from build123d import *

# Parameters (mm, degrees)
SKETCH2_W                    = 10.4902
SKETCH2_H                    = 5.7531
SKETCH3_W                    = 3.0988
SKETCH3_H                    = 1.2446
SKETCH4_R                    = 3.1496
CUT_EXTRUDE1_DEPTH           = 8.89
SKETCH5_R                    = 1
BOSS_EXTRUDE1_DEPTH          = 7.62
FILLET1_R                    = 1
SKETCH6_W                    = 2.35
SKETCH6_H                    = 0.254
SKETCH6_W_2                  = 0.254
SKETCH6_H_2                  = 2.35
EXTRUDE_THIN1_DEPTH          = 4.4958
FILLET2_R                    = 1.1
F_0_75_0_75_DIAMETER_HOLE1_D = 0.75
F_0_75_0_75_DIAMETER_HOLE2_D = 0.75
SKETCH16_OUTSIDE_W           = 23.662
SKETCH16_OUTSIDE_H           = 23.662
SKETCH16_OUTSIDE_W_2         = 11.9888
SKETCH16_OUTSIDE_H_2         = 13.0048
CUT_EXTRUDE2_DEPTH           = 9.6012


with BuildPart() as part:
    # Sketch2 → Revolve1 (revolve)
    with BuildSketch(Plane(origin=(0, 0, 0), x_dir=(0, 0, -1), z_dir=(1, 0, 0)), mode=Mode.PRIVATE) as revolve1_sk:
        with BuildLine():
            Line((-2.0066, 0), (0, 0))
            Line((0, 0), (0, 5.7531))
            Line((0, 5.7531), (0, 6.9977))
            Line((0, 6.9977), (-1.2446, 6.9977))
            ThreePointArc((-1.2446, 6.9977), (-1.783415367, 6.774515367), (-2.0066, 6.2357))
            Line((-2.0066, 6.2357), (-2.0066, 0))
        make_face()
        with Locations((5.2451, 2.87655)):
            Rectangle(SKETCH2_W, SKETCH2_H)
    revolve(revolve1_sk.sketch.rotate(Axis((0, 0, 7.880629527), (0, 0, -1)), 90), axis=Axis((0, 0, 7.880629527), (0, 0, -1)))

    # Sketch4 → Cut-Extrude1 (cut)
    with BuildSketch(Plane.XY.offset(2.0066)):
        with Locations((0, -2.4511)):
            Circle(SKETCH4_R)
    extrude(amount=-CUT_EXTRUDE1_DEPTH, mode=Mode.SUBTRACT)


with BuildPart() as body_2:
    # Sketch3 → Revolve2 (revolve)
    with BuildSketch(Plane(origin=(0, 0, 0), x_dir=(0, 0, -1), z_dir=(1, 0, 0)), mode=Mode.PRIVATE) as revolve2_sk:
        with Locations((2.4384, 6.3754)):
            Rectangle(SKETCH3_W, SKETCH3_H)
        with BuildLine():
            ThreePointArc((0, 7.62), (0.111592316, 7.889407684), (0.381, 8.001))
            Line((0.381, 8.001), (0.508, 8.001))
            ThreePointArc((0.508, 8.001), (0.777407684, 7.889407684), (0.889, 7.62))
            Line((0.889, 7.62), (0.889, 5.7531))
            Line((0.889, 5.7531), (0, 5.7531))
            Line((0, 5.7531), (0, 7.62))
        make_face()
    revolve(revolve2_sk.sketch.rotate(Axis((0, 0, 6.77031441), (0, 0, -1)), 90), axis=Axis((0, 0, 6.77031441), (0, 0, -1)))


    add(part.part)  # Boss-Extrude1 merges part
    # Sketch5 → Boss-Extrude1 (add)
    with BuildSketch(Plane.XY.offset(-6.8834)):
        with Locations(Location((0, -2.4511, 0), (0, 0, 180))):
            Circle(SKETCH5_R)
    extrude(amount=BOSS_EXTRUDE1_DEPTH)

    # Fillet1
    fillet1_edges = [body_2.edges().sort_by_distance(p)[0] for p in [
        (1, -2.4511, 0.7366),
    ]]
    fillet(fillet1_edges, radius=FILLET1_R)

    # Sketch6 → Extrude-Thin1 (add)
    with BuildSketch(Plane(origin=(0, 0, -10.4902), x_dir=(-1, 0, 0), z_dir=(0, 0, -1))):
        with Locations((0, 4.010257453)):
            Rectangle(SKETCH6_W, SKETCH6_H)
        with Locations((2.568957238, 0)):
            Rectangle(SKETCH6_W_2, SKETCH6_H_2)
    extrude(amount=EXTRUDE_THIN1_DEPTH)

    # Fillet2
    fillet2_edges = [body_2.edges().sort_by_distance(p)[0] for p in [
        (-1.175, 4.010257453, -14.986),
        (1.175, 4.010257453, -14.986),
        (-2.568957238, -1.175, -14.986),
        (-2.568957238, 1.175, -14.986),
    ]]
    fillet(fillet2_edges, radius=FILLET2_R)

    # Ø0.75 (0.75) Diameter Hole1 (through all)
    with Locations(Plane(origin=(-2.441957238, 0, 0), x_dir=(0, 0, -1), z_dir=(1, 0, 0))):
        with Locations((13.811758, 0)):
            Hole(F_0_75_0_75_DIAMETER_HOLE1_D / 2)

    # Ø0.75 (0.75) Diameter Hole2 (through all)
    with Locations(Plane(origin=(0, 4.137257453, 0), x_dir=(1, 0, 0), z_dir=(0, 1, 0))):
        with Locations((0, 13.811758)):
            Hole(F_0_75_0_75_DIAMETER_HOLE2_D / 2)

    # Sketch16 outside → Cut-Extrude2 (cut)
    with BuildSketch(Plane(origin=(0, 0, -10.4902), x_dir=(-1, 0, 0), z_dir=(0, 0, -1))):
        Rectangle(SKETCH16_OUTSIDE_W, SKETCH16_OUTSIDE_H)
        Rectangle(SKETCH16_OUTSIDE_W_2, SKETCH16_OUTSIDE_H_2, mode=Mode.SUBTRACT)
    extrude(amount=-CUT_EXTRUDE2_DEPTH, mode=Mode.SUBTRACT)


solid = body_2.part
Work out the finished part from the listing and answer in its coordinate system (mm). A direction names the side the tool comes from. Give positions to 0.01 mm unless a question says otherwise; leave off trailing zeros. Order: outer loops, then holes, each group sorted by start corner. A loop starts at its lowest first (then second) coordinate and runs counter-clockwise, first axis right, second up. Notation, with made-up numbers: M 17.25,68.5 L 46.25,68.5 A10 cw 46.25,72.5 Z; hole C -22.5,-29.5 d9. An arc over 180 degrees is marked long. Return JSON: item names as keys, results as strings.
Q1. The mould has two halves that part along Y. Classify faces 4 (the face through (6.2, 0, -0.889)), 5 (the face through (1.4, -2.4, -6.883)), 6 (the face through (0.217, -1.475, -3.62)), 7 (the face through (-1.52, 6.83, 0.63)): pulls with the +Y half, pulls with the -Y half, needs draft (parallel to the pull), parting line crosses it, or undercut.
Answer below:
{"face 4": "needs draft", "face 5": "undercut", "face 6": "undercut", "face 7": "parting line crosses it"}
Q2. Find the intervals of material crossed by line 1 along Y through (x, z) = (0, -3.75); line 2 along Z through (x, y) = (-4.75, -3.5); line 3 along Z through (x, y) = (0, 4), in increasing order. Write a range as [from, to].
Answer below:
{"line 1": "y = [-6.5, -5.6], [-3.45, -1.45], [0.7, 6.5]", "line 2": "z = [-3.99, 2.01]", "line 3": "z = [-14.99, -14.19], [-13.44, 2.01]"}
Q3. Each of these flat-tipped pins is pushed along its axis until it touches: pin 1 (8 mm diameter, centred on x = -3.5, z = -6, fed in from -Y); pin 2 (2.5 mm diameter, centred on x = -0.5, z = -3, fed in from +Y); pin 3 (0.7 mm diameter, centred on y = -0.5, z = -12, fed in from +X). Where does it stop, or does it pass through?
Answer below:
{"pin 1": "stops at y = -6.5", "pin 2": "stops at y = 6.5", "pin 3": "stops at x = -2.44"}
Q4. Which of the six approach directions +Z, -Z, +X, -X, +Y, -Y give full straight-line access (tool end or side, diameter ignored) to faces 1 (the face through (-2.696, 0, -13)), 2 (the face through (0, 4.137, -13)), 3 (the face through (-4.5, -5.36, -2.46))?
Answer below:
{"face 1": "-Z, -X, +Y, -Y", "face 2": "-Z, +X, -X, +Y", "face 3": "-Z, -X, -Y"}
Q5. Find section A-A, the plane z = -1.75. Write down the section's boundary in (x, y).
Answer below:
{"outline": "M -5.99,-3.61 A7 ccw -2.59,-6.5 L 2.59,-6.5 A7 ccw 5.99,-3.61 L 5.99,3.61 A7 ccw 2.59,6.5 L -2.59,6.5 A7 ccw -5.99,3.61 Z; C 0,-2.45 d2; hole C 0,-2.45 d6.3"}
